Here's how the part is built. I have some questions about the finished solid (model axes, mm). A direction names the side the tool comes from. Round coordinates to 2 decimals unless told otherwise and drop trailing zeros. Order: outer loops, then holes, each group sorted by start corner. A loop starts at its lowest first (then second) coordinate and runs counter-clockwise, first axis right, second up. Notation, with made-up numbers: (10.25, 21) -> (16.25, 21) arc R21 cw to (16.25, 44) -> close; hole circle Ø8 at (33.5, 52). An arc over 180 degrees is marked (long way). Answer in a Markdown table with one row per item.
```python
from build123d import *

# Parameters (mm, degrees)
SKETCH1_R           = 17.5
SKETCH1_R_2         = 3.15
BOSS_EXTRUDE1_DEPTH = 40.3
CUT_EXTRUDE1_DEPTH  = 23
CUT_EXTRUDE4_REACH  = 43.405
SKETCH8_R           = 1.65
CUT_EXTRUDE5_REACH  = 43.405
SKETCH10_R          = 1.65
SKETCH12_R          = 3
CUT_EXTRUDE6_DEPTH  = 5.35
SKETCH15_R          = 3
CUT_EXTRUDE8_DEPTH  = 5.35
CUT_EXTRUDE9_REACH  = 43.405
SKETCH17_R          = 1.65
CUT_EXTRUDE10_REACH = 43.405
SKETCH18_R          = 1.65
SKETCH19_R          = 3
CUT_EXTRUDE11_DEPTH = 5.35
CUT_EXTRUDE12_REACH = 37
SKETCH20_R          = 1.65
CUT_EXTRUDE13_REACH = 37
SKETCH21_R          = 1.65
SKETCH22_R          = 17.5
CUT_EXTRUDE14_DEPTH = 10
SKETCH23_R          = 17.5
CUT_EXTRUDE15_DEPTH = 10


with BuildPart() as part:
    # Sketch1 → Boss-Extrude1 (new body)
    with BuildSketch(Plane.XY):
        Circle(SKETCH1_R)
        Circle(SKETCH1_R_2, mode=Mode.SUBTRACT)
    extrude(amount=BOSS_EXTRUDE1_DEPTH)

    # Sketch2 → Cut-Extrude1 (cut)
    with BuildSketch(Plane.XY.offset(40.3)):
        Polygon((7.65, 0), (7.65, 2.85), (5.15, 2.85), (5.15, -2.85), (7.65, -2.85), align=None)
        Polygon((-3.825, -6.625094339), (-1.356827599, -8.050094339), (-0.106827599, -5.885030829), (-5.043172401, -3.035030829), (-6.293172401, -5.200094339), align=None)
        Polygon((-3.825, 6.625094339), (-6.293172401, 5.200094339), (-5.048242412, 3.035349353), (-0.105426694, 5.882604512), (-1.356827546, 8.050094369), align=None)
    extrude(amount=-CUT_EXTRUDE1_DEPTH, mode=Mode.SUBTRACT)

    # Sketch8 → Cut-Extrude4 (cut, up to next)
    with BuildSketch(Plane(origin=(-8.75, -15.155444566, 0), x_dir=(0, 0, -1), z_dir=(-0.5, -0.866025404, 0)), mode=Mode.PRIVATE) as cut_extrude4_sk1:
        with Locations((-20.15, 0)):
            Circle(SKETCH8_R)
    cut_extrude4_tool1 = extrude(cut_extrude4_sk1.sketch, amount=-CUT_EXTRUDE4_REACH, mode=Mode.PRIVATE) & part.part
    add(cut_extrude4_tool1.solids().sort_by_distance((-8.75, -15.155445, 20.15))[0], mode=Mode.SUBTRACT)

    # Sketch10 → Cut-Extrude5 (cut, up to next)
    with BuildSketch(Plane(origin=(-8.75, -15.155444566, 0), x_dir=(0, 0, -1), z_dir=(-0.5, -0.866025404, 0)), mode=Mode.PRIVATE) as cut_extrude5_sk1:
        with Locations((-20.15, 0)):
            Circle(SKETCH10_R)
    cut_extrude5_tool1 = extrude(cut_extrude5_sk1.sketch, amount=-CUT_EXTRUDE5_REACH, mode=Mode.PRIVATE) & part.part
    add(cut_extrude5_tool1.solids().sort_by_distance((-8.75, -15.155445, 20.15))[0], mode=Mode.SUBTRACT)

    # Sketch12 → Cut-Extrude6 (cut)
    with BuildSketch(Plane(origin=(-8.75, -15.155444566, 0), x_dir=(0, 0, -1), z_dir=(-0.5, -0.866025404, 0))):
        with Locations((-20.15, 0)):
            Circle(SKETCH12_R)
    extrude(amount=-CUT_EXTRUDE6_DEPTH, mode=Mode.SUBTRACT)

    # Sketch15 → Cut-Extrude8 (cut)
    with BuildSketch(Plane(origin=(-8.75, 15.155444566, 0), x_dir=(0, 0, -1), z_dir=(-0.5, 0.866025404, 0))):
        with Locations((-20.15, 0)):
            Circle(SKETCH15_R)
    extrude(amount=-CUT_EXTRUDE8_DEPTH, mode=Mode.SUBTRACT)

    # Sketch17 → Cut-Extrude9 (cut, up to next)
    with BuildSketch(Plane(origin=(-8.75, 15.155444566, 0), x_dir=(0, 0, -1), z_dir=(-0.5, 0.866025404, 0)), mode=Mode.PRIVATE) as cut_extrude9_sk1:
        with Locations((-20.15, 0)):
            Circle(SKETCH17_R)
    cut_extrude9_tool1 = extrude(cut_extrude9_sk1.sketch, amount=-CUT_EXTRUDE9_REACH, mode=Mode.PRIVATE) & part.part
    add(cut_extrude9_tool1.solids().sort_by_distance((-8.75, 15.155445, 20.15))[0], mode=Mode.SUBTRACT)

    # Sketch18 → Cut-Extrude10 (cut, up to next)
    with BuildSketch(Plane(origin=(-8.75, 15.155444566, 0), x_dir=(0, 0, -1), z_dir=(-0.5, 0.866025404, 0)), mode=Mode.PRIVATE) as cut_extrude10_sk1:
        with Locations((-20.15, 0)):
            Circle(SKETCH18_R)
    cut_extrude10_tool1 = extrude(cut_extrude10_sk1.sketch, amount=-CUT_EXTRUDE10_REACH, mode=Mode.PRIVATE) & part.part
    add(cut_extrude10_tool1.solids().sort_by_distance((-8.75, 15.155445, 20.15))[0], mode=Mode.SUBTRACT)

    # Sketch19 → Cut-Extrude11 (cut)
    with BuildSketch(Plane(origin=(17.5, 0, 0), x_dir=(0, 0, -1), z_dir=(1, 0, 0))):
        with Locations((-20.15, 0)):
            Circle(SKETCH19_R)
    extrude(amount=-CUT_EXTRUDE11_DEPTH, mode=Mode.SUBTRACT)

    # Sketch20 → Cut-Extrude12 (cut, up to next)
    with BuildSketch(Plane(origin=(17.5, 0, 0), x_dir=(0, 0, -1), z_dir=(1, 0, 0)), mode=Mode.PRIVATE) as cut_extrude12_sk1:
        with Locations((-20.15, 0)):
            Circle(SKETCH20_R)
    cut_extrude12_tool1 = extrude(cut_extrude12_sk1.sketch, amount=-CUT_EXTRUDE12_REACH, mode=Mode.PRIVATE) & part.part
    add(cut_extrude12_tool1.solids().sort_by_distance((17.5, 0, 20.15))[0], mode=Mode.SUBTRACT)

    # Sketch21 → Cut-Extrude13 (cut, up to next)
    with BuildSketch(Plane(origin=(17.5, 0, 0), x_dir=(0, 0, -1), z_dir=(1, 0, 0)), mode=Mode.PRIVATE) as cut_extrude13_sk1:
        with Locations((-20.15, 0)):
            Circle(SKETCH21_R)
    cut_extrude13_tool1 = extrude(cut_extrude13_sk1.sketch, amount=-CUT_EXTRUDE13_REACH, mode=Mode.PRIVATE) & part.part
    add(cut_extrude13_tool1.solids().sort_by_distance((17.5, 0, 20.15))[0], mode=Mode.SUBTRACT)

    # Sketch22 → Cut-Extrude14 (cut)
    with BuildSketch(Plane(origin=(0, 0, 0), x_dir=(-1, 0, 0), z_dir=(0, 0, -1))):
        Circle(SKETCH22_R)
    extrude(amount=-CUT_EXTRUDE14_DEPTH, mode=Mode.SUBTRACT)

    # Sketch23 → Cut-Extrude15 (cut)
    with BuildSketch(Plane.XY.offset(40.3)):
        Circle(SKETCH23_R)
    extrude(amount=-CUT_EXTRUDE15_DEPTH, mode=Mode.SUBTRACT)


solid = part.part
```
1. We'd pull the mould along X, two halves only. Please class faces 1 (the face through (-13.887, -10.648, 20.008)), 2 (the face through (14.86, -1.15, 17.38)), 3 (the face through (-0.72, 6.95, 23.89)): released by +X, released by -X, zero draft, split by the parting line, or undercut.
Numbers:
| item | result |
|---|---|
| face 1 | split by the parting line |
| face 2 | zero draft |
| face 3 | undercut |
2. Suppose I cut it at A-A on y = 0. Write out the boundary of the cut face in (x, z).
Numbers:
| item | result |
|---|---|
| outline | (-17.5, 10) -> (-3.15, 10) -> (-3.15, 30.3) -> (-17.5, 30.3) -> close; (3.15, 10) -> (17.5, 10) -> (17.5, 17.15) -> (12.15, 17.15) -> (12.15, 18.5) -> (7.65, 18.5) -> (7.65, 17.3) -> (5.15, 17.3) -> (5.15, 18.5) -> (3.15, 18.5) -> close; (3.15, 21.8) -> (5.15, 21.8) -> (5.15, 30.3) -> (3.15, 30.3) -> close; (7.65, 21.8) -> (12.15, 21.8) -> (12.15, 23.15) -> (17.5, 23.15) -> (17.5, 30.3) -> (7.65, 30.3) -> close |
3. Suppose I cut it at D-D on z = 13.75. Write out the boundary of the cut face in (x, y).
Numbers:
| item | result |
|---|---|
| outline | circle Ø35 at (0, 0); hole circle Ø6.3 at (0, 0) |
4. Suppose I cut it at B-B on z = 25.5. Write out the boundary of the cut face in (x, y) (3 decimals).
Numbers:
| item | result |
|---|---|
| outline | circle Ø35 at (0, 0); hole (-6.293, -5.2) -> (-1.357, -8.05) -> (-0.107, -5.885) -> (-5.043, -3.035) -> close; hole (-6.293, 5.2) -> (-5.048, 3.035) -> (-0.105, 5.883) -> (-1.357, 8.05) -> close; hole circle Ø6.3 at (0, 0); hole (5.15, -2.85) -> (7.65, -2.85) -> (7.65, 2.85) -> (5.15, 2.85) -> close |
5. Please list where these lines run through material, in increasing order: line 1 along Y through (x, z) = (0, 24); line 2 along Z through (x, y) = (15, 0); line 3 along X through (y, z) = (-0.5, 22).
Numbers:
| item | result |
|---|---|
| line 1 | y = -17.5 to -3.15, 3.15 to 17.5 |
| line 2 | z = 10 to 17.15, 23.15 to 30.3 |
| line 3 | x = -17.49 to -3.11, 3.11 to 5.15, 7.65 to 12.15 |
6. For faces 4 (the face through (-7.19, -9.88, 18.86)), 5 (the face through (12.15, -1.3, 18.9)), 6 (the face through (6, 0, 17.3)), 7 (the face through (0, -4, 30.3)), which set-ups out of +Z, -Z, +X, -X, +Y, -Y let a thin tool reach every point of the face, with its end or its side?
Numbers:
| item | result |
|---|---|
| face 4 | none |
| face 5 | +X |
| face 6 | +Z |
| face 7 | +Z, +X, -X, +Y, -Y |
7. Suppose I cut it at C-C on x = 4.5. Write out the boundary of the cut face in (y, z), then the cut area to 3 significant figures.
Numbers:
| item | result |
|---|---|
| outline | (-16.91, 10) -> (16.91, 10) -> (16.91, 30.3) -> (-16.91, 30.3) -> close; hole circle Ø3.3 at (0, 20.15) |
| area | 678 mm2 |
8. For pin 1 Ø8 at (y, z) = (-11, 25) entering from -X; pin 2 Ø2 at (x, z) = (6.5, 22) entering from +Y; pin 3 Ø4 at (y, z) = (9, 20.5) entering from +X, each with a flat end and sliding along its axis, tell me the tip position at first contact or that it passes through.
Numbers:
| item | result |
|---|---|
| pin 1 | stops at x = -16.04 |
| pin 2 | stops at y = 16.61 |
| pin 3 | stops at x = 16.04 |
